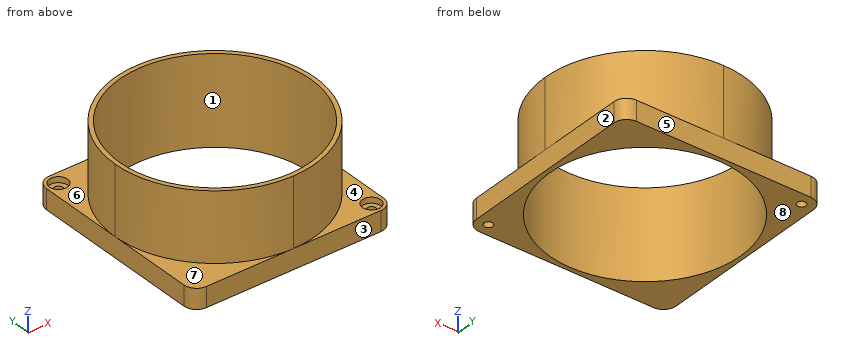
```python
from build123d import *

# Parameters (mm, degrees)
F0_R     = 33.5
F1_DEPTH = 31
F0_R_2   = 3.2
F2_DEPTH = 7
F0_R_3   = 1.5
F3_DEPTH = 5
F4_R     = 4.4


with BuildPart() as f1:
    # F0 (on Top) → F1 (new body)
    with BuildSketch(Plane.XY):
        with BuildLine():
            ThreePointArc((35, 0), (24.748737, 24.748737), (0, 35))
            ThreePointArc((0, 35), (-24.748737, 24.748737), (-35, 0))
            ThreePointArc((-35, 0), (-24.748737, -24.748737), (0, -35))
            ThreePointArc((0, -35), (24.748737, -24.748737), (35, 0))
        make_face()
        Circle(F0_R, mode=Mode.SUBTRACT)
    extrude(amount=F1_DEPTH)

    # F0 (on Top) → F2 (join)
    with BuildSketch(Plane.XY):
        with BuildLine():
            Line((35, 0), (35, 35))
            Line((35, 35), (0, 35))
            ThreePointArc((0, 35), (24.748737, 24.748737), (35, 0))
        make_face()
        with BuildLine():
            ThreePointArc((-35, 0), (-24.748737, 24.748737), (0, 35))
            Line((0, 35), (-35, 35))
            Line((-35, 35), (-35, 0))
        make_face()
        with Locations((-30.7, 30.7)):
            Circle(F0_R_2, mode=Mode.SUBTRACT)
        with BuildLine():
            Line((35, -35), (35, 0))
            ThreePointArc((35, 0), (24.748737, -24.748737), (0, -35))
            Line((0, -35), (35, -35))
        make_face()
        with Locations((30.7, -30.7)):
            Circle(F0_R_2, mode=Mode.SUBTRACT)
        with BuildLine():
            ThreePointArc((0, -35), (-24.748737, -24.748737), (-35, 0))
            Line((-35, 0), (-35, -35))
            Line((-35, -35), (0, -35))
        make_face()
    extrude(amount=F2_DEPTH)

    # F0 (on Top) → F3 (join)
    with BuildSketch(Plane.XY):
        with Locations((-30.7, 30.7)):
            Circle(F0_R_2)
        with Locations((-30.7, 30.7)):
            Circle(F0_R_3, mode=Mode.SUBTRACT)
        with Locations((30.7, -30.7)):
            Circle(F0_R_2)
        with Locations((30.7, -30.7)):
            Circle(F0_R_3, mode=Mode.SUBTRACT)
    extrude(amount=F3_DEPTH)

    # F4
    f4_edges = [f1.edges().sort_by_distance(p)[0] for p in [
        (-35, 35, 3.5),
        (35, -35, 3.5),
        (35, 35, 3.5),
        (-35, -35, 3.5),
    ]]
    fillet(f4_edges, radius=F4_R)


solid = f1.part
```
Geometry: final body of the model. Coordinates: model frame, mm. Face numbers are marked on the shaded views. A direction names the side the tool comes from. Round coordinates to 2 decimals unless told otherwise and drop trailing zeros. Write each loop counter-clockwise with the first axis right and the second up, starting at its lowest first coordinate (ties: lowest second). Pieces come first, ordered by that corner, then holes. Notation, with made-up numbers: M -31.75,20 L 21.25,20 A35 cw 21.25,59 Z; hole C 12.5,-19 d4. An arc over 180 degrees is marked long. Answer in a Markdown table with one row per item. Add a question column.
(1) Cut plane A-A, the plane z = 3. Return the cut outline in (x, y), then the cut area to 3 significant figures.
(2) Reachability of the marked faces 4, 5, 6, 7 and 8 from +Z, -Z, +X, -X, +Y, -Y: full face, straight path, thin tool, end or side. Return the list, or none.
(3) Cut plane C-C, the plane z = 19. Return the cut outline in (x, y).
(4) Cut plane B-B, the plane y = 25. Return the cut outline in (x, z), then the cut area to 3 significant figures.
(5) Ray query, L1, parallel to Y at x = 30, z = 3; L2, parallel to Y at x = 30, z = 6; L3, parallel to Y at x = 0, z = 9. Return the intervals inside material, ascending.
(6) Cut plane D-D, the plane x = -17.5. Return the cut outline in (y, z).
(7) Draft query along Y for the marked faces 1, 2 and 3. Return one class per face: pulls with the +Y half, pulls with the -Y half, needs draft (parallel to the pull), parting line crosses it, or undercut.
(8) Contact query for flat-ended pins moving along their axis: pin 1 (4 mm diameter, centred on x = -30.7, y = 30.7, fed in from +Z); pin 2 (8 mm diameter, centred on x = -0.5, z = 8.5, fed in from -Y); pin 3 (4 mm diameter, centred on x = 7, z = 25, fed in from -Y); pin 4 (1 mm diameter, centred on y = -15, z = 21.5, fed in from -X). Output: stop coordinate, or through.
Established:
| question | item | result |
|---|---|---|
| 1 | outline | M -35,-30.6 A4.4 ccw -30.6,-35 L 30.6,-35 A4.4 ccw 35,-30.6 L 35,30.6 A4.4 ccw 30.6,35 L -30.6,35 A4.4 ccw -35,30.6 Z; hole C 0,0 d67; hole C -30.7,30.7 d3; hole C 30.7,-30.7 d3 |
| 1 | area | 1,340 mm² |
| 2 | face 4 | +Z, +X, -Y |
| 2 | face 5 | +Z, -Z, +X, -X, +Y |
| 2 | face 6 | +Z, -X, +Y |
| 2 | face 7 | +Z, -X, -Y |
| 2 | face 8 | -Z, +X, -X, +Y, -Y |
| 3 | outline | M -35,0 A35 ccw 0,-35 A35 ccw 35,0 A35 ccw 0,35 A35 ccw Z; hole C 0,0 d67 |
| 4 | outline | M -35,0 L -22.3,0 L -22.3,31 L -24.49,31 L -24.49,7 L -35,7 Z; M 22.3,0 L 35,0 L 35,7 L 24.49,7 L 24.49,31 L 22.3,31 Z |
| 4 | area | 283 mm² |
| 5 | L1 | -35 to -32.03, -29.37 to -14.91, 14.91 to 35 |
| 5 | L2 | -35 to -33.82, -27.58 to -14.91, 14.91 to 35 |
| 5 | L3 | -35 to -33.5, 33.5 to 35 |
| 6 | outline | M -35,0 L -28.57,0 L -28.57,31 L -30.31,31 L -30.31,7 L -35,7 Z; M 28.57,0 L 35,0 L 35,7 L 30.31,7 L 30.31,31 L 28.57,31 Z |
| 7 | face 1 | undercut |
| 7 | face 2 | needs draft |
| 7 | face 3 | pulls with the -Y half |
| 8 | pin 1 | z = 5 |
| 8 | pin 2 | y = -35 |
| 8 | pin 3 | y = -34.64 |
| 8 | pin 4 | x = -31.86 |
